Part model, mm, in its own coordinate system. A direction names the side the tool comes from. Give positions to 0.01 mm unless a question says otherwise; leave off trailing zeros. Order: outer loops, then holes, each group sorted by start corner. A loop starts at its lowest first (then second) coordinate and runs counter-clockwise, first axis right, second up. Notation, with made-up numbers: M 51,52.25 L 95,52.25 A6 ccw 95,59.25 Z; hole C 3,72 d11. An arc over 180 degrees is marked long. Return JSON: item names as keys, results as strings.
from build123d import *

# Parameters (mm, degrees)
PAD_DEPTH    = 12.7
CHAMFER_SIZE = 1


with BuildPart() as part:
    # Sketch → Pad (new body)
    with BuildSketch(Plane.XY):
        Polygon((-6.35, 0), (-6.35, 4.2164), (0, 4.2164), (0, 1.6764), (-2.38125, 1.6764), (-2.38125, 0), align=None)
    extrude(amount=PAD_DEPTH)

    # Chamfer
    chamfer_edges = [part.edges().sort_by_distance(p)[0] for p in [
        (0, 1.6764, 6.35),
    ]]
    chamfer(chamfer_edges, length=CHAMFER_SIZE)


solid = part.part
Q1. Band-saw the part on C-C (y = 1.2). Give the cut face in (x, z).
Established:
{"outline": "M -6.35,0 L -2.38,0 L -2.38,12.7 L -6.35,12.7 Z"}
Q2. Two-plate mould, pull along X, no slides. Class faces 3 (the flat face through (-4, 2, 0)), 4 (the flat face through (-0.507, 2.169, 6.261)), 5 (the flat face through (-6.35, 2, 6)): +X half, -X half, draft (parallel to the pull), parting line (faces both ways), or undercut.
Established:
{"face 3": "draft", "face 4": "+X half", "face 5": "-X half"}
Q3. Band-saw the part on A-A (z = 8.5). Give the cut face in (x, y).
Established:
{"outline": "M -6.35,0 L -2.38,0 L -2.38,1.68 L -1,1.68 L 0,2.68 L 0,4.22 L -6.35,4.22 Z"}
Q4. Probe line 1 along X through (y, z) = (0.9, 8.75); line 2 along Y through (x, z) = (-2.25, 6.25); line 3 along X through (y, z) = (2.05, 7.75). List the from-to ranges inside material, lowest first.
Established:
{"line 1": "x = -6.35 to -2.38", "line 2": "y = 1.68 to 4.22", "line 3": "x = -6.35 to -0.63"}
Q5. Pin check, flat tip, straight feed: pin 1 (0.5 mm diameter, centred on y = 1, z = 8.5, fed in from +X). Stop position of the tip, or through.
Established:
{"pin 1": "stops at x = -2.38"}
Q6. Band-saw the part on B-B (x = -1.25). Give the cut face in (y, z), then the cut area to 3 significant figures.
Established:
{"outline": "M 1.68,0 L 4.22,0 L 4.22,12.7 L 1.68,12.7 Z", "area": "32.3 mm²"}
Q7. 3-axis set-ups, long thin cutter, end or side, ignore diameter. For faces 1 (the flat face through (-2, 1.676, 6)), 2 (the flat face through (-3, 4.216, 6)): which of +Z, -Z, +X, -X, +Y, -Y reach the whole face in a straight line?
Established:
{"face 1": "+Z, -Z, +X, -Y", "face 2": "+Z, -Z, +X, -X, +Y"}
